```python
from build123d import *

# Parameters (mm, degrees)
SKETCH3_W               = 56.4388
SKETCH3_H               = 112.8776
SKETCH3_W_2             = 9.4615
SKETCH3_H_2             = 56.4388
CUT_EXTRUDE1_DEPTH      = 15.875
HOLE1_D                 = 9.525
HOLE1_DEPTH             = 20.955
HOLE1_TIP               = 2.749630657
SKETCH8_R               = 4.38785
CUT_EXTRUDE2_DEPTH      = 7.096125
CUT_EXTRUDE2_DEPTH_BACK = 7.096125


with BuildPart() as part:
    # Sketch1 → Revolve1 (revolve)
    with BuildSketch(Plane.XY):
        Polygon((0, 0), (0, 12.84605), (0.762, 13.60805), (4.826, 13.60805), (5.588, 12.84605), (6.35, 12.84605), (6.35, 14.1097), (21.463, 14.1097), (22.225, 13.3477), (22.225, 0), align=None)
    revolve(axis=Axis((22.225, 0, 0), (-1, 0, 0)))

    # Sketch2 → Revolve2 (revolve)
    with BuildSketch(Plane.XY):
        with BuildLine():
            Line((22.225, 0), (22.225, 7.90575))
            Line((22.225, 7.90575), (24.6126, 7.90575))
            Line((24.6126, 7.90575), (24.6126, 7.72795))
            ThreePointArc((24.6126, 7.72795), (24.872982072, 7.099332072), (25.5016, 6.83895))
            Line((25.5016, 6.83895), (26.7843, 6.83895))
            ThreePointArc((26.7843, 6.83895), (27.10530348, 6.898927826), (27.38299292, 7.0707683))
            Line((27.38299292, 7.0707683), (27.412917928, 7.09803))
            Line((27.412917928, 7.09803), (28.252387928, 7.9375))
            Line((28.252387928, 7.9375), (37.26053, 7.9375))
            Line((37.26053, 7.9375), (38.1, 7.09803))
            Line((38.1, 7.09803), (38.1, 0))
            Line((38.1, 0), (22.225, 0))
        make_face()
    revolve(axis=Axis((38.1, 0, 0), (-1, 0, 0)))

    # Sketch3 → Cut-Extrude1 (cut)
    with BuildSketch(Plane(origin=(38.1, 0, 0), x_dir=(0, 0, -1), z_dir=(1, 0, 0))):
        Rectangle(SKETCH3_W, SKETCH3_H)
        Rectangle(SKETCH3_W_2, SKETCH3_H_2, mode=Mode.SUBTRACT)
    extrude(amount=-CUT_EXTRUDE1_DEPTH, mode=Mode.SUBTRACT)

    # Hole1
    with Locations(Plane.ZY):
        with Locations((0, 0)):
            Hole(HOLE1_D / 2, depth=HOLE1_DEPTH)
            with Locations((0, 0, -(HOLE1_DEPTH + HOLE1_TIP / 2))):  # 120° drill point
                Cone(0, HOLE1_D / 2, HOLE1_TIP, mode=Mode.SUBTRACT)

    # Sketch6 → Cut-Revolve1 (revolve, cut)
    with BuildSketch(Plane(origin=(0, 0, 0), x_dir=(1, 0, 0), z_dir=(0, 0.999847695, 0.017452406))):
        Polygon((15.0876, 0), (19.710593378, 0), (19.710593378, -7.1755), (19.927075925, -14.1097), (15.0876, -14.1097), align=None)
    revolve(axis=Axis((15.0876, -0.246248219, 14.107551024), (0, 0.017452406, -0.999847695)), mode=Mode.SUBTRACT)

    # Sketch7 → Revolve3 (revolve)
    with BuildSketch(Plane.XY):
        with BuildLine():
            Line((5.48614893, 14.025531804), (6.227512806, 13.284167928))
            ThreePointArc((6.227512806, 13.284167928), (6.264710245, 13.194365367), (6.227512806, 13.104562806))
            Line((6.227512806, 13.104562806), (5.969, 12.84605))
            Line((5.969, 12.84605), (5.588, 12.84605))
            Line((5.588, 12.84605), (5.588, 12.59205))
            Line((5.588, 12.59205), (6.35, 12.59205))
            Line((6.35, 12.59205), (6.35, 13.44904893))
            Line((6.35, 13.44904893), (5.68934893, 14.1097))
            Line((5.68934893, 14.1097), (5.48614893, 14.1097))
            Line((5.48614893, 14.1097), (5.48614893, 14.025531804))
        make_face()
    revolve(axis=Axis((6.35, 0, 0), (-1, 0, 0)))

    # Sketch8 → Cut-Extrude2 (cut, two sides)
    with BuildSketch(Plane.XY) as cut_extrude2_sk:
        with Locations((30.9626, 0)):
            Circle(SKETCH8_R)
    extrude(amount=CUT_EXTRUDE2_DEPTH, mode=Mode.SUBTRACT)
    extrude(cut_extrude2_sk.sketch, amount=-CUT_EXTRUDE2_DEPTH_BACK, mode=Mode.SUBTRACT)


solid = part.part
```
Work out the finished part from the listing and answer in its coordinate system (mm). A direction names the side the tool comes from. Round coordinates to 2 decimals unless told otherwise and drop trailing zeros. Loops run counter-clockwise (first coordinate to the right, second up) from the corner with the lowest first, then second, coordinate; pieces in that order, holes last.
(1) For faces 1 (the cylindrical face through (26.15, 6.84, 0.07)), 2 (the cylindrical face through (2.82, 12.57, 5.21)), determine the directions among +Z, -Z, +X, -X, +Y, -Y from which every point of the face is accessible in a straight line to the end or side of a thin tool.
Computed values:
face 1: +Y
face 2: -X
(2) The part is cut by section A-A, the plane x = 34. Give the vertices of the cut face in (y, z) (1 decimal), and give its area (3 significant figures).
Computed values:
outline: (-6.4, -4.7) - (-3.2, -4.7) - (-3.2, 4.7) - (-6.4, 4.7) arc R7.9 ccw to start; (3.2, -4.7) - (6.4, -4.7) arc R7.9 ccw to (6.4, 4.7) - (3.2, 4.7) - close
area: 80.8 mm2
(3) The part is cut by section B-B, the plane x = 20.5. Give the vertices of the cut face in (y, z) (1 decimal), and give its area (3 significant figures).
Computed values:
outline: circle Ø28.2 at (0, 0); hole circle Ø9.5 at (0, 0)
area: 554 mm2
(4) Each of these flat-tipped pins is pushed along its axis until it touches: P1, Ø10, axis at x = 29.5, y = 1.5, coming from the -Z side; P2, Ø3, axis at y = -9.5, z = 9.5, coming from the +X side (3 decimals); P3, Ø6.5, axis at x = 28.5, y = 2, coming from the +Z side. Where does it stop, or does it pass through?
Computed values:
P1: stops at z = -4.73
P2: stops at x = 22.225
P3: stops at z = 4.73
(5) Find the intervals of material crossed by L1, parallel to Z at x = 8.75, y = 0; L2, parallel to Z at x = 27, y = -2.5, in increasing order.
Computed values:
L1: z = -14.11 to -4.76, 4.76 to 14.11
L2: z = -4.73 to 4.73
(6) The part is cut by section C-C, the plane y = -2. Give the number of separate pieces and of enclosed holes in the cut face, and give its area (3 significant figures).
Computed values:
separate pieces: 3
enclosed holes: 0
area: 415 mm2
(7) The mould has two halves that part along Y. Classify faces 3 (the cylindrical face through (10.624, 1.431, -4.543)), 4 (the conical face through (17.271, 4.012, 10.763)), 5 (the cylindrical face through (32.82, 7.937, 0.071)), 6 (the flat face through (0, -6, 0)): pulls with the +Y half, pulls with the -Y half, needs draft (parallel to the pull), parting line crosses it, or undercut.
Computed values:
face 3: undercut
face 4: undercut
face 5: pulls with the +Y half
face 6: needs draft
